Part model, mm, in its own coordinate system. A direction names the side the tool comes from. Give positions to 0.01 mm unless a question says otherwise; leave off trailing zeros. Order: outer loops, then holes, each group sorted by start corner. A loop starts at its lowest first (then second) coordinate and runs counter-clockwise, first axis right, second up. Notation, with made-up numbers: M 70,47.25 L 124,47.25 A29 ccw 124,73.25 Z; hole C 24.25,40.25 d8. An arc over 180 degrees is marked long. Answer as a JSON object with one key per item and string values.
from build123d import *

# Parameters (mm, degrees)
F1_DEPTH = 2
F2_DEPTH = 2


with BuildPart() as f1:
    # F0 (on Top) → F1 (new body, symmetric)
    with BuildSketch(Plane.XY):
        with BuildLine():
            ThreePointArc((4.25, -5), (3.5855613229, -7.2817208418), (1.8, -8.85))
            Line((1.8, -8.85), (1.8, -16.2))
            Line((1.8, -16.2), (10.1, -16.2))
            Line((10.1, -16.2), (11.2, -14.2))
            Line((11.2, -14.2), (10.1, -14.2))
            Line((10.1, -14.2), (10.1, -13))
            Line((10.1, -13), (14, -13))
            Line((14, -13), (14, -10))
            Line((14, -10), (7.25, -10))
            Line((7.25, -10), (7.25, -5))
            Line((7.25, -5), (7.25, -2.5))
            Line((7.25, -2.5), (7.25, 0))
            ThreePointArc((7.25, 0), (5.1265241636, 5.1265241636), (0, 7.25))
            ThreePointArc((0, 7.25), (-5.1265241636, 5.1265241636), (-7.25, 0))
            Line((-7.25, 0), (-7.25, -2.5))
            Line((-7.25, -2.5), (-7.25, -5))
            Line((-7.25, -5), (-7.25, -10))
            Line((-7.25, -10), (-14, -10))
            Line((-14, -10), (-14, -13))
            Line((-14, -13), (-10.1, -13))
            Line((-10.1, -13), (-10.1, -14.2))
            Line((-10.1, -14.2), (-11.2, -14.2))
            Line((-11.2, -14.2), (-10.1, -16.2))
            Line((-10.1, -16.2), (-1.8, -16.2))
            Line((-1.8, -16.2), (-1.8, -8.85))
            ThreePointArc((-1.8, -8.85), (-3.5855613229, -7.2817208418), (-4.25, -5))
            Line((-4.25, -5), (-4.25, -2.5))
            Line((-4.25, -2.5), (-4.25, 0))
            ThreePointArc((-4.25, 0), (-3.00520382, 3.00520382), (0, 4.25))
            ThreePointArc((0, 4.25), (3.00520382, 3.00520382), (4.25, 0))
            Line((4.25, 0), (4.25, -2.5))
            Line((4.25, -2.5), (4.25, -5))
        make_face()
    extrude(amount=F1_DEPTH, both=True)

    # F0 (on Top) → F2 (join)
    with BuildSketch(Plane.XY):
        with BuildLine():
            ThreePointArc((0, 2.75), (2.6185133227, 0.8401713984), (1.6, -2.2366269246))
            Line((1.6, -2.2366269246), (1.6, -3.0790627288))
            ThreePointArc((1.6, -3.0790627288), (2.4962673742, -4.8634379387), (1.8, -6.7349351573))
            Line((1.8, -6.7349351573), (1.8, -8.85))
            ThreePointArc((1.8, -8.85), (3.5855613229, -7.2817208418), (4.25, -5))
            Line((4.25, -5), (4.25, -2.5))
            Line((4.25, -2.5), (4.25, 0))
            ThreePointArc((4.25, 0), (3.00520382, 3.00520382), (0, 4.25))
            ThreePointArc((0, 4.25), (-3.00520382, 3.00520382), (-4.25, 0))
            Line((-4.25, 0), (-4.25, -2.5))
            Line((-4.25, -2.5), (-4.25, -5))
            ThreePointArc((-4.25, -5), (-3.5855613229, -7.2817208418), (-1.8, -8.85))
            Line((-1.8, -8.85), (-1.8, -6.7349351573))
            ThreePointArc((-1.8, -6.7349351573), (-2.4962673742, -4.8634379387), (-1.6, -3.0790627288))
            Line((-1.6, -3.0790627288), (-1.6, -2.2366269246))
            ThreePointArc((-1.6, -2.2366269246), (-2.6185133227, 0.8401713984), (0, 2.75))
        make_face()
    extrude(amount=F2_DEPTH)


solid = f1.part
1. Which spindle directions (+Z, -Z, +X, -X, +Y, -Y) get a long thin tool onto all of the face, cutting with end or side? Do faces 4 (the flat face through (-4.25, -3, -1)), 5 (the flat face through (7.25, -5, 0)), 6 (the flat face through (-11, -14.2, 0)), 7 (the flat face through (11, -14.2, 0)). Say none if no direction does.
Worked answers:
{"face 4": "-Z", "face 5": "+Z, -Z, +X, +Y", "face 6": "+Z, -Z, -X", "face 7": "+Z, -Z, +X"}
2. Pin check, flat tips, straight feed: P1, Ø0.6, axis at y = -2.5, z = -1, coming from the +X side; P2, Ø1.2, axis at x = -11, z = 0, coming from the +Y side; P3, Ø1, axis at y = -14, z = 0.5, coming from the -X side. Stop position of each tip, or through.
Worked answers:
{"P1": "stops at x = 7.25", "P2": "stops at y = -10", "P3": "stops at x = -11.2"}
3. Cut at D-D on x = -7.75. Give the cut face in (y, z).
Worked answers:
{"outline": "M -16.2,-2 L -10,-2 L -10,2 L -16.2,2 Z"}
4. Probe line 1 along X through (y, z) = (-9, 1.4); line 2 along X through (y, z) = (-13.25, -0.25); line 3 along Y through (x, z) = (8.25, -0.05). List the from-to ranges inside material, lowest first.
Worked answers:
{"line 1": "x = -7.25 to -1.8, 1.8 to 7.25", "line 2": "x = -10.1 to -1.8, 1.8 to 10.1", "line 3": "y = -16.2 to -10"}
5. Cut at A-A on y = -3.5. Give the cut face in (x, z), plus the area to 3 significant figures.
Worked answers:
{"outline": "M -7.25,-2 L -4.25,-2 L -4.25,0 L -2,0 L -2,2 L -7.25,2 Z; M 2,0 L 4.25,0 L 4.25,-2 L 7.25,-2 L 7.25,2 L 2,2 Z", "area": "33.0 mm^2"}
6. Two-plate mould, pull along X, no slides. Class faces 1 (the flat face through (6, -16.2, 0)), 2 (the flat face through (-7.25, -5, 0)), 3 (the cylindrical face through (3.604, -7.253, -0.986)): +X half, -X half, draft (parallel to the pull), parting line (faces both ways), or undercut.
Worked answers:
{"face 1": "draft", "face 2": "-X half", "face 3": "undercut"}
7. Cut at B-B on z = 1. Give the cut face in (x, y).
Worked answers:
{"outline": "M -14,-13 L -10.1,-13 L -10.1,-14.2 L -11.2,-14.2 L -10.1,-16.2 L -1.8,-16.2 L -1.8,-6.73 A2.5 cw -1.6,-3.08 L -1.6,-2.24 A2.75 cw long 1.6,-2.24 L 1.6,-3.08 A2.5 cw 1.8,-6.73 L 1.8,-16.2 L 10.1,-16.2 L 11.2,-14.2 L 10.1,-14.2 L 10.1,-13 L 14,-13 L 14,-10 L 7.25,-10 L 7.25,0 A7.25 ccw -7.25,0 L -7.25,-10 L -14,-10 Z"}
8. Cut at C-C on y = -8.5. Give the cut face in (x, z), plus the area to 3 significant figures.
Worked answers:
{"outline": "M -7.25,-2 L -2.41,-2 L -2.41,0 L -1.8,0 L -1.8,2 L -7.25,2 Z; M 1.8,0 L 2.41,0 L 2.41,-2 L 7.25,-2 L 7.25,2 L 1.8,2 Z", "area": "41.2 mm^2"}
